Can you work these out from the model? Positions are in its coordinate system, mm. A direction names the side the tool comes from. Round coordinates to 2 decimals unless told otherwise and drop trailing zeros. Write each loop counter-clockwise with the first axis right and the second up, starting at its lowest first coordinate (ties: lowest second). Pieces come first, ordered by that corner, then holes. Notation, with made-up numbers: (-22, 72) - (-17, 72) arc R18 cw to (-17, 90) - close; hole circle Ø10 at (2, 44.5). An arc over 180 degrees is marked (long way). One line per item, written item: value. Start each with the question number.
(1) I'm going to push flat-ended pins straight in: pin 1 Ø8 at (x, y) = (-59.5, -59.5) entering from +Z; pin 2 Ø0.9 at (x, z) = (-59, 2) entering from +Y; pin 3 Ø0.9 at (y, z) = (-58.5, 1.5) entering from -X; pin 4 Ø5 at (x, y) = (-12.5, 7) entering from -Z. Where does each tip first touch, or does it pass through?
(2) I want a section at A-A on y = -30. List the corners of the cut face in (x, z) for me, plus the area to 3 significant figures.
(3) On a 3-axis mill with a long thin cutter (end or side, diameter ignored), from which of +Z, -Z, +X, -X, +Y, -Y can I reach the whole of each face in a straight line? I mean faces 1 (the face through (-70, 55.5, 11)), 2 (the face through (-55.5, -70, 11)), 3 (the face through (70, 55.5, 11)). Say none if no direction works.
(4) Thinking about a two-plate mould opening in Y: for faces 4 (the face through (64.07, 64, 1.52)), 5 (the face through (1, -69, 14)), 6 (the face through (-1, 1, 0)), 7 (the face through (64, -64.07, 1.52)), which applies, +Y half, -Y half, draft (parallel to the pull), parting line (faces both ways), or undercut?
(5) I want a section at B-B on z = 7.75. List the corners of the cut face in (x, y) for me.
(6) If I drill on L1, parallel to Y at x = 59.5, z = 2.2; L2, parallel to Y at x = -48.5, z = 10.5, over which ranges is the centre line in solid material (lowest first)? Write a range as from..to.
(7) I want a section at C-C on y = 30. List the corners of the cut face in (x, z) for me, plus the area to 3 significant figures.
Autodesk Inventor part; units mm, degrees
ref_plane "YZ Plane" through (0, 0, 0) normal (1, 0, 0) x (0, 1, 0)
ref_plane "XZ Plane" through (0, 0, 0) normal (0, 1, 0) x (-1, 0, 0)
ref_plane "XY Plane" through (0, 0, 0) normal (0, 0, 1) x (1, 0, 0)
sketch "Sketch1" plane through (0, 0, 0) normal (0, 0, 1) x (1, 0, 0)
  line L0 (55.5, 72) -> (-55.5, 72)
  line L1 (-55.5, 72) -> (-55.5, 65.5)
  line L2 (-55.5, 65.5) -> (-65.5, 65.5)
  line L3 (-65.5, 65.5) -> (-65.5, 55.5)
  line L4 (-65.5, 55.5) -> (-72, 55.5)
  line L5 (-72, 55.5) -> (-72, -55.5)
  line L6 (-72, -55.5) -> (-65.5, -55.5)
  line L7 (-65.5, -55.5) -> (-65.5, -65.5)
  line L8 (-65.5, -65.5) -> (-55.5, -65.5)
  line L9 (-55.5, -65.5) -> (-55.5, -72)
  line L10 (-55.5, -72) -> (55.5, -72)
  line L11 (55.5, -72) -> (55.5, -65.5)
  line L12 (55.5, -65.5) -> (65.5, -65.5)
  line L13 (65.5, -65.5) -> (65.5, -55.5)
  line L14 (65.5, -55.5) -> (72, -55.5)
  line L15 (72, -55.5) -> (72, 55.5)
  line L16 (72, 55.5) -> (65.5, 55.5)
  line L17 (65.5, 55.5) -> (65.5, 65.5)
  line L18 (65.5, 65.5) -> (55.5, 65.5)
  line L19 (55.5, 65.5) -> (55.5, 72)
  point P0 (0, 0)
  dimension "d5" = 144
  dimension "d14" = 144
  dimension "d15" = 72
  dimension "d16" = 72
  dimension "d28" = 10
  dimension "d30" = 10
  dimension "d31" = 10
  dimension "d32" = 111
  dimension "d33" = 111
extrude "Plate1" add sketch "Sketch1" along normal blind 3
sketch "Sketch2" plane through (-69, -55.5, 0) normal (-1, 0, 0) x (0, -1, 0)
  line L0 (-111, 0) -> (0, 0)
  line L1 (0, 0) -> (0, 22.5)
  line L2 (0, 22.5) -> (-111, 22.5)
  line L3 (-111, 22.5) -> (-111, 0)
edge flange "Flange1" height 22.5 angle 90 thickness 3 bend radius 3 thickness toward (-1, 0, 0) relief tear relief width 3 relief depth 0 corner gap 3 corner form 0 edges at (-72, 0, 3) (0, -72, 3) (72, 0, 3) (0, 72, 3) wall of the first edge with corners at (-69, 55.5, 0) (-69, -55.5, 0) (-69, -55.5, 22.5) (-69, 55.5, 22.5)
bend "Bend1"
corner "Corner1"
sketch "Sketch3" plane through (0, 0, 3) normal (0, 0, 1) x (1, 0, 0)
  line L0 (59.5, -59.5) -> (-59.5, -59.5)
  line L1 (-59.5, -59.5) -> (-59.5, 59.5)
  line L2 (-59.5, 59.5) -> (59.5, 59.5)
  line L3 (59.5, 59.5) -> (59.5, -59.5)
  circle A0 centre (59.5, -59.5) radius 3
  point P0 (0, 0)
  dimension "d34" = 119
  dimension "d35" = 119
  dimension "d36" = 59.5
  dimension "d37" = 59.5
  dimension "d38" = 6
hole "Hole1" at (59.5, -59.5, 3) at (-59.5, -59.5, 3) at (-59.5, 59.5, 3) at (59.5, 59.5, 3) direction (0, 0, -1) diameter 4.917 end through all
fillet "Corner Round1" radius 5 4 edges at (65.5, -65.5, 1.5) (65.5, 65.5, 1.5) (-65.5, 65.5, 1.5) (-65.5, -65.5, 1.5)
sketch "Sketch4" plane through (0, 0, 3) normal (0, 0, 1) x (1, 0, 0)
  line L0 (45, -25) -> (25, -25)
  line L1 (25, -25) -> (25, -40)
  line L2 (25, -40) -> (45, -40)
  line L3 (45, -40) -> (45, -25)
  point P0 (0, 0)
  dimension "d47" = 20
  dimension "d48" = 15
  dimension "d49" = 25
  dimension "d50" = 25
extrude "Cut1" cut sketch "Sketch4" against normal blind 3
equation "\"d40\" = Thickness"
equation "\"d44\" = Thickness"
equation "\"d51\" = Thickness"
equation "\"d17\" = Thickness"
equation "\"d18\" = BendReliefWidth"
equation "\"d20\" = MinimumRemnant"
equation "\"d21\" = TransitionRadius"
equation "\"d24\" = BendRadius"
equation "\"d25\" = CornerReliefSize"
equation "\"d26\" = GapSize"
equation "\"d27\" = JacobiRadiusSize"
equation "\"BendRadius\" = Thickness"
equation "\"BendReliefWidth\" = Thickness"
equation "\"BendReliefDepth\" = 0.5 * Thickness"
equation "\"CornerReliefSize\" = 4 * Thickness"
equation "\"MinimumRemnant\" = 2 * Thickness"
equation "\"TransitionRadius\" = BendRadius"
equation "\"JacobiRadiusSize\" = BendRadius"
equation "\"GapSize\" = Thickness"
properties part number "WaageBlechUnterseite"
Established:
1. pin 1: z = 3
1. pin 2: y = 65.5
1. pin 3: x = -65.5
1. pin 4: z = 0
2. outline: (-72, 6) arc R6 ccw to (-66, 0) - (25, 0) - (25, 3) - (-66, 3) arc R3 cw to (-69, 6) - (-69, 22.5) - (-72, 22.5) - close; (45, 0) - (66, 0) arc R6 ccw to (72, 6) - (72, 22.5) - (69, 22.5) - (69, 6) arc R3 cw to (66, 3) - (45, 3) - close
2. area: 477 mm2
3. face 1: +Z, -Z, -X, +Y
3. face 2: +Z, -Z, -X, -Y
3. face 3: +Z, -Z, +X, +Y
4. face 4: +Y half
4. face 5: undercut
4. face 6: draft
4. face 7: -Y half
5. outline: (-72, -55.5) - (-69, -55.5) - (-69, 55.5) - (-72, 55.5) - close; (-55.5, -72) - (55.5, -72) - (55.5, -69) - (-55.5, -69) - close; (-55.5, 69) - (55.5, 69) - (55.5, 72) - (-55.5, 72) - close; (69, -55.5) - (72, -55.5) - (72, 55.5) - (69, 55.5) - close
6. L1: -65.5..-61.96, -57.04..57.04, 61.96..65.5
6. L2: -72..-69, 69..72
7. outline: (-72, 6) arc R6 ccw to (-66, 0) - (66, 0) arc R6 ccw to (72, 6) - (72, 22.5) - (69, 22.5) - (69, 6) arc R3 cw to (66, 3) - (-66, 3) arc R3 cw to (-69, 6) - (-69, 22.5) - (-72, 22.5) - close
7. area: 537 mm2
